from build123d import *

# Parameters (mm, degrees)
SKETCH2_W             = 86.37
SKETCH2_H             = 30
BOSS_EXTRUDE1_DEPTH   = 1.5875
F_1_CLEARANCE_HOLE1_D = 2.2606
F_6_CLEARANCE_HOLE1_D = 3.7973


with BuildPart() as part:
    # Sketch2 → Boss-Extrude1 (new body)
    with BuildSketch(Plane.XY):
        with Locations((0, 15)):
            Rectangle(SKETCH2_W, SKETCH2_H)
    extrude(amount=BOSS_EXTRUDE1_DEPTH)

    # #1 Clearance Hole1 (through all)
    with Locations(Plane.XY.offset(1.5875)):
        with Locations((35.185, 23.2), (35.185, 5), (-35.185, 5), (-35.185, 23.2)):
            Hole(F_1_CLEARANCE_HOLE1_D / 2)

    # #6 Clearance Hole1 (through all)
    with Locations(Plane(origin=(0, 0, 0), x_dir=(-1, 0, 0), z_dir=(0, 0, -1))):
        with Locations((7.5, 15), (-7.5, 15)):
            Hole(F_6_CLEARANCE_HOLE1_D / 2)


solid = part.part
Design review of the part built by this model. Coordinates are the model's own, in mm. Give positions to 0.01 mm unless a question says otherwise; leave off trailing zeros. Write each loop counter-clockwise with the first axis right and the second up, starting at its lowest first coordinate (ties: lowest second). Pieces come first, ordered by that corner, then holes. Notation, with made-up numbers: M -24,-3.5 L -15,-3.5 A34 ccw -15,26.5 Z; hole C 32.25,-17.5 d6. An arc over 180 degrees is marked long. Return JSON: item names as keys, results as strings. Group by question number.
Item 1: The part is to be moulded in two halves that separate along X. For faces 1 (the cylindrical face through (36.08, 4.31, 0.78)), 2 (the flat face through (-1, 30, 1)), 3 (the flat face through (43.185, 15, 1)), say which applies: pulls with the +X half, pulls with the -X half, needs draft (parallel to the pull), parting line crosses it, or undercut.
Item 2: Wall thickness on line 1 along X through (y, z) = (16.25, 0.75) (3 decimals); line 2 along X through (y, z) = (23.5, 1.4) (3 decimals); line 3 along Y through (x, z) = (-7.5, 0.7): over which ranges is each line inside the solid? List them lowest first.
Item 3: Take a section at A-A (y = 23.2). Give the boundary of the cut face in (x, z) (1 decimal).
Item 4: Take a section at C-C (y = 15). Give the boundary of the cut face in (x, z) (1 decimal), plus the area to 3 significant figures.
Item 5: Take a section at B-B (x = -7.5). Give the boundary of the cut face in (y, z).
Item 6: Clearance check with a flat-ended pin moving along its axis: pin 1 Ø2 at (x, y) = (35.185, 23.2) entering from -Z. State where the tip first meets the part, or that it passes through.
Return value:
{
 "1": {"face 1": "undercut", "face 2": "needs draft", "face 3": "pulls with the +X half"},
 "2": {"line 1": "x = -43.185 to -8.929, -6.071 to 6.071, 8.929 to 43.185", "line 2": "x = -43.185 to -36.275, -34.095 to 34.095, 36.275 to 43.185", "line 3": "y = 0 to 13.1, 16.9 to 30"},
 "3": {"outline": "M -43.2,0 L -36.3,0 L -36.3,1.6 L -43.2,1.6 Z; M -34.1,0 L 34.1,0 L 34.1,1.6 L -34.1,1.6 Z; M 36.3,0 L 43.2,0 L 43.2,1.6 L 36.3,1.6 Z"},
 "4": {"outline": "M -43.2,0 L -9.4,0 L -9.4,1.6 L -43.2,1.6 Z; M -5.6,0 L 5.6,0 L 5.6,1.6 L -5.6,1.6 Z; M 9.4,0 L 43.2,0 L 43.2,1.6 L 9.4,1.6 Z", "area": "125 mm2"},
 "5": {"outline": "M 0,0 L 13.1,0 L 13.1,1.59 L 0,1.59 Z; M 16.9,0 L 30,0 L 30,1.59 L 16.9,1.59 Z"},
 "6": {"pin 1": "passes through"}
}
